The drawing under review shows one solid part. Ordinate dimensions are in mm from its lowest x, y, z. Coordinates: 2 decimals unless noted, no trailing zeros. Loops run counter-clockwise (first coordinate to the right, second up) from the corner with the lowest first, then second, coordinate; pieces in that order, holes last. Notation, with made-up numbers: M -34,60 L -17,60 A16 ccw -17,87 Z; hole C 48,53.25 d1. An arc over 180 degrees is marked long. Use one line per item in the form item = value.
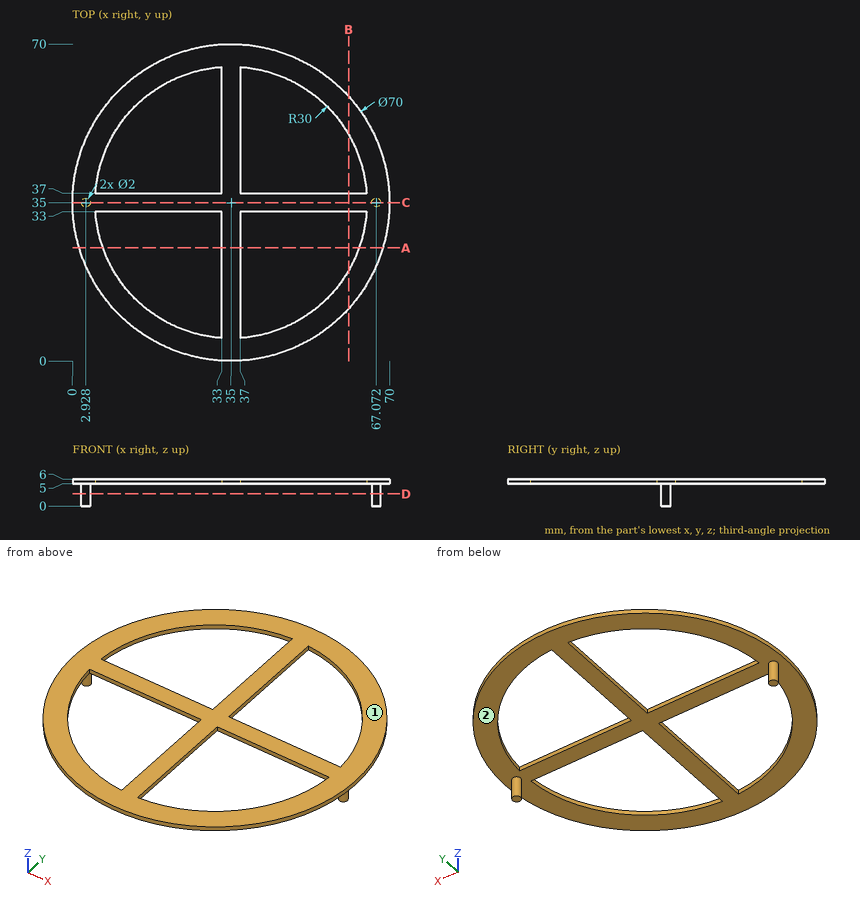
1. Consider section B-B on x = 61. Write out the cut boundary in (y, z).
Computed values:
outline = M 11.57,5 L 20.03,5 L 20.03,6 L 11.57,6 Z; M 33,5 L 37,5 L 37,6 L 33,6 Z; M 49.97,5 L 58.43,5 L 58.43,6 L 49.97,6 Z
2. Consider section A-A on y = 25. Write out the cut boundary in (x, z).
Computed values:
outline = M 1.46,5 L 6.72,5 L 6.72,6 L 1.46,6 Z; M 33,5 L 37,5 L 37,6 L 33,6 Z; M 63.28,5 L 68.54,5 L 68.54,6 L 63.28,6 Z
3. Consider section C-C on y = 35. Write out the cut boundary in (x, z), plus the area to 3 significant figures.
Computed values:
outline = M 0,5 L 1.93,5 L 1.93,0 L 3.93,0 L 3.93,5 L 66.07,5 L 66.07,0 L 68.07,0 L 68.07,5 L 70,5 L 70,6 L 0,6 Z
area = 90.0 mm2
4. Wall thickness on line 1 along Z through (x, y) = (37, 5): over which ranges is the line inside the solid? List them lowest first. Write a range as from..to.
Computed values:
line_1 = 5..6
5. For pin 1 Ø0.5 at (y, z) = (20.5, 5.5) entering from +X; pin 2 Ø2 at (x, z) = (45.5, 3.5) entering from -Y; pin 3 Ø1.1 at (y, z) = (50.5, 5.5) entering from -X; pin 4 Ø0.5 at (y, z) = (47.5, 5.5) entering from +X, all flat-tipped, find the tip position at first contact; note any pin that passes through.
Computed values:
pin_1 = 66.97
pin_2 = through
pin_3 = 3.35
pin_4 = 67.79
6. Draft analysis for pull direction X (two halves, no side actions). For the marked faces 1 and 2, state which applies: +X half, -X half, draft (parallel to the pull), parting line (faces both ways), or undercut.
Computed values:
face_1 = draft
face_2 = undercut
7. Consider section D-D on z = 2.7. Write out the cut boundary in (x, y).
Computed values:
outline = C 2.93,35 d2; C 67.07,35 d2
